from build123d import *

# Parameters (mm, degrees)
F0_W     = 3
F0_H     = 3
F1_DEPTH = 4


with BuildPart() as f1:
    # F0 (on Front) → F1 (new body, symmetric)
    with BuildSketch(Plane.XZ):
        Polygon((-33.5, 0), (-47, 0), (-47, -2.5), (-44, -2.5), (-36, -2.5), (-36, -17.5), (0, -17.5), (0, -15), (-33.5, -15), align=None)
        with Locations((-45.5, -4)):
            Rectangle(F0_W, F0_H)
    extrude(amount=F1_DEPTH, both=True)

    # F3: F1 across plane


with BuildPart() as f1_1:
    add(f1.part)
    add(f1.part.mirror(Plane.YZ))


solid = f1_1.part
Input: part model. Units: mm. Frame: model coordinates. A direction names the side the tool comes from. Give positions to 0.01 mm unless a question says otherwise; leave off trailing zeros. Loops run counter-clockwise (first coordinate to the right, second up) from the corner with the lowest first, then second, coordinate; pieces in that order, holes last. Notation, with made-up numbers: (45, 63) - (89, 63) arc R11 ccw to (89, 67) - close; hole circle Ø11 at (33, -15). An arc over 180 degrees is marked (long way). Use CSV: the item, a comma, the result in double quotes. Start each with the question number.
Item 1: Section D-D on x = -15. Return loops of the section in (y, z).
Item 2: Line query: line 1 (X direction, y = -3.5, z = -4); line 2 (X direction, y = 0.5, z = -12.5); line 3 (Z direction, x = -26, y = 3.25). Output: solid intervals per line, ascending.
Item 3: Section A-A on z = -1.5. Return loops of the section in (x, y), then the cut area to 3 significant figures.
Item 4: Contact query for flat-ended pins moving along their axis: P1, Ø2.5, axis at y = 1, z = -6.5, coming from the +X side; P2, Ø2.5, axis at y = -0.5, z = -9.5, coming from the -X side; P3, Ø2.5, axis at y = 0.5, z = -10.5, coming from the +X side; P4, Ø2.5, axis at x = 45, y = 1, coming from the -Z side. Output: stop coordinate, or through.
Item 5: Section C-C on z = -9.5. Return loops of the section in (x, y).
Item 6: Reachability of faces 4 (the flat face through (-46, 0, -5.5)), 5 (the flat face through (-36, 0, -10)), 6 (the flat face through (-40, 0, 0)), 7 (the flat face through (-33.5, 0, -8)) from +Z, -Z, +X, -X, +Y, -Y: full face, straight path, thin tool, end or side. Return the list, or none.
Item 7: Mould query, pull axis X, two halves, no side actions, for faces 1 (the flat face through (47, 0, -3)), 2 (the flat face through (46, 0, -5.5)), 3 (the flat face through (40, 0, -2.5)). Classes: pulls with the +X half, pulls with the -X half, needs draft (parallel to the pull), parting line crosses it, or undercut.
Item 8: Section B-B on y = 1.75. Return loops of the section in (x, z).
Ans:
1,outline,"(-4, -17.5) - (4, -17.5) - (4, -15) - (-4, -15) - close"
2,line 1,"x = -47 to -44, -36 to -33.5, 33.5 to 36, 44 to 47"
2,line 2,"x = -36 to -33.5, 33.5 to 36"
2,line 3,"z = -17.5 to -15"
3,outline,"(-47, -4) - (-33.5, -4) - (-33.5, 4) - (-47, 4) - close; (33.5, -4) - (47, -4) - (47, 4) - (33.5, 4) - close"
3,area,"216 mm2"
4,P1,"stops at x = 47"
4,P2,"stops at x = -36"
4,P3,"stops at x = 36"
4,P4,"stops at z = -5.5"
5,outline,"(-36, -4) - (-33.5, -4) - (-33.5, 4) - (-36, 4) - close; (33.5, -4) - (36, -4) - (36, 4) - (33.5, 4) - close"
6,face 4,"-Z, -X, +Y, -Y"
6,face 5,"-Z, +Y, -Y"
6,face 6,"+Z, +X, -X, +Y, -Y"
6,face 7,"+Z, +Y, -Y"
7,face 1,"pulls with the +X half"
7,face 2,"needs draft"
7,face 3,"undercut"
8,outline,"(-47, -5.5) - (-44, -5.5) - (-44, -2.5) - (-36, -2.5) - (-36, -17.5) - (36, -17.5) - (36, -2.5) - (44, -2.5) - (44, -5.5) - (47, -5.5) - (47, 0) - (33.5, 0) - (33.5, -15) - (-33.5, -15) - (-33.5, 0) - (-47, 0) - close"
